```python
from build123d import *

# Parameters (mm, degrees)
F0_W     = 254
F0_H     = 127
F0_R     = 25.4
F1_DEPTH = 127
F2_W     = 25.4
F2_H     = 38.1
F3_DEPTH = 76.2
F4_R     = 7.62
F5_R     = 5.08


with BuildPart() as f1:
    # F0 (on Front) → F1 (new body)
    with BuildSketch(Plane.XZ):
        with Locations((127, 63.5)):
            Rectangle(F0_W, F0_H)
        with Locations((177.8, 63.5)):
            Circle(F0_R, mode=Mode.SUBTRACT)
    extrude(amount=F1_DEPTH)

    # F2 (on face) → F3 (join)
    with BuildSketch(Plane.XZ.offset(127)):
        with Locations((63.5, 44.45)):
            Rectangle(F2_W, F2_H)
    extrude(amount=F3_DEPTH)

    # F4
    f4_edges = [f1.edges().sort_by_distance(p)[0] for p in [
        (254, -127, 63.5),
    ]]
    fillet(f4_edges, radius=F4_R)

    # F5
    f5_edges = [f1.edges().sort_by_distance(p)[0] for p in [
        (254, -59.69, 0),
        (251.768154, -124.768154, 0),
        (127, 0, 0),
        (123.19, -127, 0),
        (0, -63.5, 0),
        (0, -127, 63.5),
        (123.19, -127, 127),
    ]]
    fillet(f5_edges, radius=F5_R)


solid = f1.part
```
Geometry: final body of the model. Coordinates: model frame, mm. A direction names the side the tool comes from. Round coordinates to 2 decimals unless told otherwise and drop trailing zeros. Order: outer loops, then holes, each group sorted by start corner. A loop starts at its lowest first (then second) coordinate and runs counter-clockwise, first axis right, second up. Notation, with made-up numbers: (82, -21.5) -> (137, -21.5) arc R16 cw to (137, -0.5) -> close; hole circle Ø8 at (5, -1.5). An arc over 180 degrees is marked (long way). Use one line per item in the form item = value. Start each with the question number.
1. Draft query along Z for faces 4 (the face through (201.263, -62.611, 53.772)), 5 (the face through (50.8, -165, 44)), 6 (the face through (63, -165, 25.4)). Return one class per face: pulls with the +Z half, pulls with the -Z half, needs draft (parallel to the pull), parting line crosses it, or undercut.
2. Pin query (flat end, axial travel): pin 1 Ø8 at (x, z) = (178.5, 114) entering from -Y; pin 2 Ø19 at (y, z) = (-160, 45.5) entering from -X; pin 3 Ø7.5 at (x, y) = (67, -156) entering from +Z. Return the tip coordinate at first contact, or that it passes through.
3. Cut plane A-A (y = -89). Return the cut outline in (x, z).
4. Cut plane D-D (z = 21). Return the cut outline in (x, y), then the cut area to 3 significant figures.
5. Cut plane C-C (x = 123.5). Return the cut outline in (y, z), then the cut area to 3 significant figures.
6. Line query: probe 1 along Z at (x, y) = (177, -59); probe 2 along Y at (x, z) = (217, 56); probe 3 along Z at (x, y) = (184.5, -99). Output: solid intervals per line, ascending.
7. Reachability of faces 1 (the face through (125, -63, 0)), 2 (the face through (76.2, -165, 44)), 3 (the face through (63, -165, 63.5)) from +Z, -Z, +X, -X, +Y, -Y: full face, straight path, thin tool, end or side. Return the list, or none.
8. Cut plane B-B (x = 177.8). Return the cut outline in (y, z).
Solution:
q1.face_4 = undercut
q1.face_5 = needs draft
q1.face_6 = pulls with the -Z half
q2.pin_1 = -127
q2.pin_2 = 50.8
q2.pin_3 = 63.5
q3.outline = (0, 5.08) arc R5.08 ccw to (5.08, 0) -> (248.92, 0) arc R5.08 ccw to (254, 5.08) -> (254, 121.92) arc R5.08 ccw to (248.92, 127) -> (0, 127) -> close; hole circle Ø50.8 at (177.8, 63.5)
q4.outline = (0, -121.92) arc R5.08 ccw to (5.08, -127) -> (246.38, -127) arc R7.62 ccw to (254, -119.38) -> (254, 0) -> (0, 0) -> close
q4.area = 32,200 mm^2
q5.outline = (-127, 5.08) arc R5.08 ccw to (-121.92, 0) -> (-5.08, 0) arc R5.08 ccw to (0, 5.08) -> (0, 127) -> (-121.92, 127) arc R5.08 ccw to (-127, 121.92) -> close
q5.area = 16,100 mm^2
q6.probe_1 = 0 to 38.11, 88.89 to 127
q6.probe_2 = -127 to 0
q6.probe_3 = 0 to 39, 88 to 127
q7.face_1 = -Z, +X, -X, +Y, -Y
q7.face_2 = +Z, -Z, +X, -Y
q7.face_3 = +Z, +X, -X, -Y
q8.outline = (-127, 5.08) arc R5.08 ccw to (-121.92, 0) -> (-5.08, 0) arc R5.08 ccw to (0, 5.08) -> (0, 38.1) -> (-127, 38.1) -> close; (-127, 88.9) -> (0, 88.9) -> (0, 127) -> (-121.92, 127) arc R5.08 ccw to (-127, 121.92) -> close
